The model under review builds one solid part; all positions refer to its coordinate system, in mm. A direction names the side the tool comes from. Coordinates: 2 decimals unless noted, no trailing zeros. Loops run counter-clockwise (first coordinate to the right, second up) from the corner with the lowest first, then second, coordinate; pieces in that order, holes last. Notation, with made-up numbers: (-29, 17.5) - (-23, 17.5) arc R15 cw to (-23, 21.5) - close; hole circle Ø10 at (57.25, 20.25). An arc over 180 degrees is marked (long way). Use a Markdown table: item, result. Add a question column.
1) To check wall thickness, follow L1, parallel to Z at x = 4, y = 1.1; L2, parallel to X at y = 6.75, z = 1.5; L3, parallel to Y at x = 4, z = 0.8. State the ranges of each line that lie inside material, in increasing order. Write a range as [from, to].
2) Clearance check with flat-ended pins moving along their axes: pin 1 (1.8 mm diameter, centred on x = 4, z = 4, fed in from +Y); pin 2 (6 mm diameter, centred on x = 17, y = 7.5, fed in from +Z); pin 3 (1.5 mm diameter, centred on x = 11, z = 4, fed in from +Y). State where each tip first meets the part, or that it passes through.
3) The part is to be moulded in two halves that separate along Y. For faces 3 (the cylindrical face through (5.43, 1.01, 3.55)), 4 (the cylindrical face through (5.386, 6.425, 1.014)), 5 (the flat face through (10, 0, 4)), 6 (the cylindrical face through (14.8, 6.1, 1)), say which applies: pulls with the +Y half, pulls with the -Y half, needs draft (parallel to the pull), parting line crosses it, or undercut.
4) Add section D-D, the plane y = 1.75. Give the boundary of the cut face in (x, z), and give its area (3 significant figures).
5) Add section A-A, the plane x = 16. Give the boundary of the cut face in (y, z), and give its area (3 significant figures).
6) Add section B-B, the plane z = 4. Give the boundary of the cut face in (x, y).
7) For faces 1 (the flat face through (10, 2, 4)), 2 (the flat face through (0, 4, 1)), list the 3-axis set-ups (+Z, -Z, +X, -X, +Y, -Y) from which the entire face can be reached by the end or side of a thin tool; tool diameter is ignored.
```python
from build123d import *

# Parameters (mm, degrees)
RESSALTO_EXTRUS_O1_DEPTH = 20
ESBO_O2_R                = 1.5
CORTE_EXTRUS_O1_DEPTH    = 3
ESBO_O3_R                = 1.5
CORTE_EXTRUS_O2_DEPTH    = 3


with BuildPart() as part:
    # Esboço1 → Ressalto-extrusão1 (new body)
    with BuildSketch(Plane(origin=(0, 0, 0), x_dir=(0, 0, -1), z_dir=(1, 0, 0))):
        Polygon((0, 0), (0, 10), (-2, 10), (-2, 2), (-7, 2), (-7, 0), align=None)
    extrude(amount=RESSALTO_EXTRUS_O1_DEPTH)

    # Esboço2 → Corte-extrusão1 (cut, through all)
    with BuildSketch(Plane(origin=(0, 2, 0), x_dir=(1, 0, 0), z_dir=(0, 1, 0))):
        with Locations((4, -4)):
            Circle(ESBO_O2_R)
        with Locations((16, -4)):
            Circle(ESBO_O2_R)
    extrude(amount=-CORTE_EXTRUS_O1_DEPTH, mode=Mode.SUBTRACT)

    # Esboço3 → Corte-extrusão2 (cut, through all)
    with BuildSketch(Plane.XY.offset(2)):
        with Locations((4, 7)):
            Circle(ESBO_O3_R)
        with Locations((16, 7)):
            Circle(ESBO_O3_R)
    extrude(amount=-CORTE_EXTRUS_O2_DEPTH, mode=Mode.SUBTRACT)


solid = part.part
```
From the geometry:
| question | item | result |
|---|---|---|
| 1 | L1 | z = [0, 2.5], [5.5, 7] |
| 1 | L2 | x = [0, 2.52], [5.48, 14.52], [17.48, 20] |
| 1 | L3 | y = [0, 5.5], [8.5, 10] |
| 2 | pin 1 | passes through |
| 2 | pin 2 | stops at z = 2 |
| 2 | pin 3 | stops at y = 2 |
| 3 | face 3 | needs draft |
| 3 | face 4 | undercut |
| 3 | face 5 | pulls with the -Y half |
| 3 | face 6 | undercut |
| 4 | outline | (0, 0) - (20, 0) - (20, 7) - (0, 7) - close; hole circle Ø3 at (4, 4); hole circle Ø3 at (16, 4) |
| 4 | area | 126 mm^2 |
| 5 | outline | (0, 0) - (5.5, 0) - (5.5, 2) - (2, 2) - (2, 2.5) - (0, 2.5) - close; (0, 5.5) - (2, 5.5) - (2, 7) - (0, 7) - close; (8.5, 0) - (10, 0) - (10, 2) - (8.5, 2) - close |
| 5 | area | 18.0 mm^2 |
| 6 | outline | (0, 0) - (2.5, 0) - (2.5, 2) - (0, 2) - close; (5.5, 0) - (14.5, 0) - (14.5, 2) - (5.5, 2) - close; (17.5, 0) - (20, 0) - (20, 2) - (17.5, 2) - close |
| 7 | face 1 | +Z, +X, -X, +Y |
| 7 | face 2 | +Z, -Z, -X, +Y, -Y |
